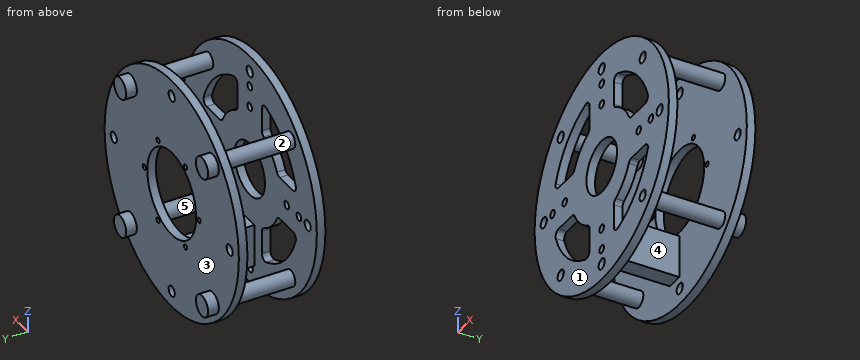
```python
from build123d import *

# Parameters (mm, degrees)
SKETCH1_R           = 139.7
SKETCH1_R_2         = 31.75
SKETCH1_R_3         = 6.35
SKETCH1_R_4         = 4.699
BOSS_EXTRUDE1_DEPTH = 10.16
SKETCH2_R           = 9.525
BOSS_EXTRUDE2_DEPTH = 82.296
SKETCH3_R           = 139.7
SKETCH3_R_2         = 50.8
SKETCH3_R_3         = 6.35
SKETCH3_R_4         = 3.175
BOSS_EXTRUDE3_DEPTH = 10.16
SKETCH4_R           = 12.7
BOSS_EXTRUDE4_DEPTH = 12.7
SKETCH6_W           = 19.812
SKETCH6_H           = 50.8
BOSS_EXTRUDE5_DEPTH = 76.2


with BuildPart() as part:
    # Sketch1 → Boss-Extrude1 (new body)
    with BuildSketch(Plane(origin=(0, 0, 0), x_dir=(1, 0, 0), z_dir=(0, 1, 0))):
        Circle(SKETCH1_R)
        Circle(SKETCH1_R_2, mode=Mode.SUBTRACT)
        with Locations((0, 120.65)):
            Circle(SKETCH1_R_3, mode=Mode.SUBTRACT)
        with Locations((0, 102.362)):
            Circle(SKETCH1_R_4, mode=Mode.SUBTRACT)
        with Locations((0, 76.962)):
            Circle(SKETCH1_R_4, mode=Mode.SUBTRACT)
        with Locations((85.31243315, 85.31243315)):
            Circle(SKETCH1_R_3, mode=Mode.SUBTRACT)
        with Locations((120.65, 0)):
            Circle(SKETCH1_R_3, mode=Mode.SUBTRACT)
        with Locations((85.31243315, -85.31243315)):
            Circle(SKETCH1_R_3, mode=Mode.SUBTRACT)
        with Locations((0, -120.65)):
            Circle(SKETCH1_R_3, mode=Mode.SUBTRACT)
        with Locations((-85.31243315, -85.31243315)):
            Circle(SKETCH1_R_3, mode=Mode.SUBTRACT)
        with Locations((-120.65, 0)):
            Circle(SKETCH1_R_3, mode=Mode.SUBTRACT)
        with Locations((-85.31243315, 85.31243315)):
            Circle(SKETCH1_R_3, mode=Mode.SUBTRACT)
        with Locations((102.362, 0)):
            Circle(SKETCH1_R_4, mode=Mode.SUBTRACT)
        with Locations((76.962, 0)):
            Circle(SKETCH1_R_4, mode=Mode.SUBTRACT)
        with Locations((0, -102.362)):
            Circle(SKETCH1_R_4, mode=Mode.SUBTRACT)
        with Locations((0, -76.962)):
            Circle(SKETCH1_R_4, mode=Mode.SUBTRACT)
        with Locations((-102.362, 0)):
            Circle(SKETCH1_R_4, mode=Mode.SUBTRACT)
        with Locations((-76.962, 0)):
            Circle(SKETCH1_R_4, mode=Mode.SUBTRACT)
        with BuildLine():
            Line((-25.4, 89.802561211), (-25.4, 62.217039467))
            ThreePointArc((-25.4, 62.217039467), (-26.334701805, 58.900860121), (-28.863636364, 56.56094497))
            ThreePointArc((-28.863636364, 56.56094497), (-44.901280605, 44.901280605), (-56.56094497, 28.863636364))
            ThreePointArc((-56.56094497, 28.863636364), (-58.900860121, 26.334701805), (-62.217039467, 25.4))
            Line((-62.217039467, 25.4), (-89.802561211, 25.4))
            ThreePointArc((-89.802561211, 25.4), (-94.9873145, 28.083825791), (-95.789398625, 33.866666667))
            ThreePointArc((-95.789398625, 33.866666667), (-71.842048969, 71.842048969), (-33.866666667, 95.789398625))
            ThreePointArc((-33.866666667, 95.789398625), (-28.083825791, 94.9873145), (-25.4, 89.802561211))
        make_face(mode=Mode.SUBTRACT)
        with BuildLine():
            Line((25.4, 89.802561211), (25.4, 62.217039467))
            ThreePointArc((25.4, 62.217039467), (26.334701805, 58.900860121), (28.863636364, 56.56094497))
            ThreePointArc((28.863636364, 56.56094497), (44.901280605, 44.901280605), (56.56094497, 28.863636364))
            ThreePointArc((56.56094497, 28.863636364), (58.900860121, 26.334701805), (62.217039467, 25.4))
            Line((62.217039467, 25.4), (89.802561211, 25.4))
            ThreePointArc((89.802561211, 25.4), (94.9873145, 28.083825791), (95.789398625, 33.866666667))
            ThreePointArc((95.789398625, 33.866666667), (71.842048969, 71.842048969), (33.866666667, 95.789398625))
            ThreePointArc((33.866666667, 95.789398625), (28.083825791, 94.9873145), (25.4, 89.802561211))
        make_face(mode=Mode.SUBTRACT)
        with BuildLine():
            Line((89.802561211, -25.4), (62.217039467, -25.4))
            ThreePointArc((62.217039467, -25.4), (58.900860121, -26.334701805), (56.56094497, -28.863636364))
            ThreePointArc((56.56094497, -28.863636364), (44.901280605, -44.901280605), (28.863636364, -56.56094497))
            ThreePointArc((28.863636364, -56.56094497), (26.334701805, -58.900860121), (25.4, -62.217039467))
            Line((25.4, -62.217039467), (25.4, -89.802561211))
            ThreePointArc((25.4, -89.802561211), (28.083825791, -94.9873145), (33.866666667, -95.789398625))
            ThreePointArc((33.866666667, -95.789398625), (71.842048969, -71.842048969), (95.789398625, -33.866666667))
            ThreePointArc((95.789398625, -33.866666667), (94.9873145, -28.083825791), (89.802561211, -25.4))
        make_face(mode=Mode.SUBTRACT)
        with BuildLine():
            Line((-25.4, -89.802561211), (-25.4, -62.217039467))
            ThreePointArc((-25.4, -62.217039467), (-26.334701805, -58.900860121), (-28.863636364, -56.56094497))
            ThreePointArc((-28.863636364, -56.56094497), (-44.901280605, -44.901280605), (-56.56094497, -28.863636364))
            ThreePointArc((-56.56094497, -28.863636364), (-58.900860121, -26.334701805), (-62.217039467, -25.4))
            Line((-62.217039467, -25.4), (-89.802561211, -25.4))
            ThreePointArc((-89.802561211, -25.4), (-94.9873145, -28.083825791), (-95.789398625, -33.866666667))
            ThreePointArc((-95.789398625, -33.866666667), (-71.842048969, -71.842048969), (-33.866666667, -95.789398625))
            ThreePointArc((-33.866666667, -95.789398625), (-28.083825791, -94.9873145), (-25.4, -89.802561211))
        make_face(mode=Mode.SUBTRACT)
    extrude(amount=BOSS_EXTRUDE1_DEPTH)

    # Sketch2 → Boss-Extrude2 (add)
    with BuildSketch(Plane(origin=(0, 10.16, 0), x_dir=(1, 0, 0), z_dir=(0, 1, 0))):
        with Locations((-85.31243315, 85.31243315)):
            Circle(SKETCH2_R)
        with Locations((85.31243315, 85.31243315)):
            Circle(SKETCH2_R)
        with Locations((85.31243315, -85.31243315)):
            Circle(SKETCH2_R)
        with Locations((-85.31243315, -85.31243315)):
            Circle(SKETCH2_R)
    extrude(amount=BOSS_EXTRUDE2_DEPTH)

    # Sketch3 → Boss-Extrude3 (add)
    with BuildSketch(Plane(origin=(0, 92.456, 0), x_dir=(1, 0, 0), z_dir=(0, 1, 0))):
        Circle(SKETCH3_R)
        Circle(SKETCH3_R_2, mode=Mode.SUBTRACT)
        with Locations((0, 120.65)):
            Circle(SKETCH3_R_3, mode=Mode.SUBTRACT)
        with Locations((85.31243315, 85.31243315)):
            Circle(SKETCH3_R_3, mode=Mode.SUBTRACT)
        with Locations((120.65, 0)):
            Circle(SKETCH3_R_3, mode=Mode.SUBTRACT)
        with Locations((85.31243315, -85.31243315)):
            Circle(SKETCH3_R_3, mode=Mode.SUBTRACT)
        with Locations((0, -120.65)):
            Circle(SKETCH3_R_3, mode=Mode.SUBTRACT)
        with Locations((-85.31243315, -85.31243315)):
            Circle(SKETCH3_R_3, mode=Mode.SUBTRACT)
        with Locations((-120.65, 0)):
            Circle(SKETCH3_R_3, mode=Mode.SUBTRACT)
        with Locations((-85.31243315, 85.31243315)):
            Circle(SKETCH3_R_3, mode=Mode.SUBTRACT)
        with Locations((-57.15, 0)):
            Circle(SKETCH3_R_4, mode=Mode.SUBTRACT)
        with Locations((-28.575, 49.493351826)):
            Circle(SKETCH3_R_4, mode=Mode.SUBTRACT)
        with Locations((28.575, 49.493351826)):
            Circle(SKETCH3_R_4, mode=Mode.SUBTRACT)
        with Locations((57.15, 0)):
            Circle(SKETCH3_R_4, mode=Mode.SUBTRACT)
        with Locations((28.575, -49.493351826)):
            Circle(SKETCH3_R_4, mode=Mode.SUBTRACT)
        with Locations((-28.575, -49.493351826)):
            Circle(SKETCH3_R_4, mode=Mode.SUBTRACT)
    extrude(amount=BOSS_EXTRUDE3_DEPTH)

    # Sketch4 → Boss-Extrude4 (add)
    with BuildSketch(Plane(origin=(0, 102.616, 0), x_dir=(1, 0, 0), z_dir=(0, 1, 0))):
        with Locations((-85.31243315, 85.31243315)):
            Circle(SKETCH4_R)
        with Locations((85.31243315, 85.31243315)):
            Circle(SKETCH4_R)
        with Locations((85.31243315, -85.31243315)):
            Circle(SKETCH4_R)
        with Locations((-85.31243315, -85.31243315)):
            Circle(SKETCH4_R)
    extrude(amount=BOSS_EXTRUDE4_DEPTH)

    # Sketch6 → Boss-Extrude5 (add)
    with BuildSketch(Plane(origin=(0, 10.16, 0), x_dir=(1, 0, 0), z_dir=(0, 1, 0))):
        with Locations((0, 88.9)):
            Rectangle(SKETCH6_W, SKETCH6_H)
    extrude(amount=BOSS_EXTRUDE5_DEPTH)


solid = part.part
```
Work out the finished part from the listing and answer in its coordinate system (mm). Face numbers are marked on the shaded views. A direction names the side the tool comes from. Coordinates: 2 decimals unless noted, no trailing zeros. Loops run counter-clockwise (first coordinate to the right, second up) from the corner with the lowest first, then second, coordinate; pieces in that order, holes last. Notation, with made-up numbers: M 4.5,10 L 12.5,10 A25 cw 12.5,27 Z; hole C 49.25,66.25 d7. An arc over 180 degrees is marked long. Use CSV: the item, a comma, the result in double quotes. Start each with the question number.
(1) Find section B-B, the plane x = 120.65. Give the vertices of the cut face in (y, z).
(2) For the marked faces 4 and 5, determine the directions among +Z, -Z, +X, -X, +Y, -Y from which every point of the face is accessible in a straight line to the end or side of a thin tool.
(3) Given pin 1 Ø10 at (x, z) = (0, -120.65) entering from +Y; pin 2 Ø3 at (x, y) = (75, 74.5) entering from +Z; pin 3 Ø11 at (y, z) = (6.5, -80) entering from -X; pin 4 Ø6 at (x, z) = (-19.5, -61.5) entering from +Y, each flat-ended and moving along its own axis, determine where each tip first touches the part or whether it passes through.
(4) Find section C-C, the plane y = 47.5. Give the vertices of the cut face in (x, z) (3 decimals).
(5) For a pull along Y with two mould halves and no side action, classify the marked faces 1, 2 and 3 as +Y half, -Y half, draft (parallel to the pull), parting line (faces both ways), or undercut.
(6) Consider line 1 (Y direction, x = -57, z = 100.5); line 2 (Y direction, x = 83.5, z = -46); line 3 (X direction, y = 4, z = 120). Determine where each line is inside the solid, lowest interval first.
(7) Find section A-A, the plane z = -14.5. Give the vertices of the cut face in (x, y), then the cut area to 3 significant figures.
Recorded:
1,outline,"M 0,-70.42 L 10.16,-70.42 L 10.16,-6.35 L 0,-6.35 Z; M 0,6.35 L 10.16,6.35 L 10.16,70.42 L 0,70.42 Z; M 92.46,-70.42 L 102.62,-70.42 L 102.62,-6.35 L 92.46,-6.35 Z; M 92.46,6.35 L 102.62,6.35 L 102.62,70.42 L 92.46,70.42 Z"
2,face 4,"+Z, -Z"
2,face 5,"none"
3,pin 1,"passes through"
3,pin 2,"stops at z = 88.93"
3,pin 3,"stops at x = -118.18"
3,pin 4,"stops at y = 102.62"
4,outline,"C -85.312,-85.312 d19.05; C -85.312,85.312 d19.05; M -9.906,-114.3 L 9.906,-114.3 L 9.906,-63.5 L -9.906,-63.5 Z; C 85.312,-85.312 d19.05; C 85.312,85.312 d19.05"
5,face 1,"-Y half"
5,face 2,"undercut"
5,face 3,"+Y half"
6,line 1,"y = 0 to 10.16, 92.46 to 102.62"
6,line 2,"y = 92.46 to 102.62"
6,line 3,"x = -71.53 to -6.32, 6.32 to 71.53"
7,outline,"M -138.95,0 L -28.25,0 L -28.25,10.16 L -138.95,10.16 Z; M -138.95,92.46 L -48.69,92.46 L -48.69,102.62 L -138.95,102.62 Z; M 28.25,0 L 138.95,0 L 138.95,10.16 L 28.25,10.16 Z; M 48.69,92.46 L 138.95,92.46 L 138.95,102.62 L 48.69,102.62 Z"
7,area,"4,080 mm^2"
